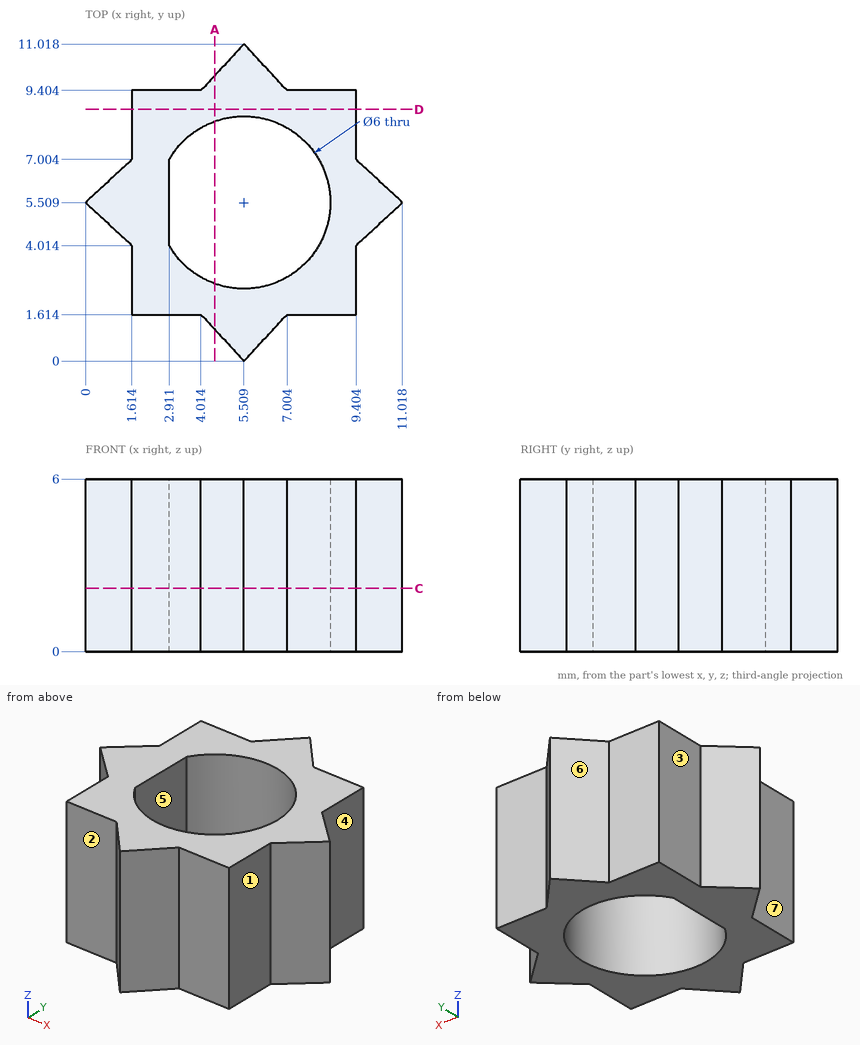
Drawing for the job (mm, zero at the part's lowest x, y, z). A direction names the side the tool comes from. Give positions to 0.01 mm unless a question says otherwise; leave off trailing zeros. Order: outer loops, then holes, each group sorted by start corner. A loop starts at its lowest first (then second) coordinate and runs counter-clockwise, first axis right, second up. Notation, with made-up numbers: (-12, 28.5) - (17, 28.5) arc R7 cw to (17, 34.5) - close; hole circle Ø1 at (56, 73.5). An arc over 180 degrees is marked (long way). Write item = value, one per line. Start each with the question number.
1. Drop flat-ended pins along their axis: P1, Ø2, axis at y = 6, z = 4, coming from the -X side; P2, Ø0.7, axis at y = 3.5, z = 2.5, coming from the -X side; P3, Ø1.9, axis at x = 2.5, z = 1.5, coming from the +Y side (1 decimal); P4, Ø1.9, axis at y = 8.5, z = 4.5, coming from the +X side (1 decimal). Give the stop position or say it passes through.
2. Probe line 1 along Y through (x, z) = (9, 4.6) (1 decimal); line 2 along X through (y, z) = (3.5, 2.75) (1 decimal); line 3 along X through (y, z) = (7.5, 4.55) (1 decimal). List the from-to ranges inside material, lowest first.
3. Cut at D-D, the plane y = 8.75. List the corners of the cut face in (x, z) (1 decimal).
4. Which spindle directions (+Z, -Z, +X, -X, +Y, -Y) get a long thin tool onto all of the face, cutting with end or side? Do the marked faces 1, 2, 3 and 4. Say none if no direction does.
5. Cut at A-A, the plane x = 4.5. List the corners of the cut face in (y, z) (1 decimal).
6. Two-plate mould, pull along Y, no slides. Class the marked faces 5, 6 and 7: pulls with the +Y half, pulls with the -Y half, needs draft (parallel to the pull), parting line crosses it, or undercut.
7. Cut at C-C, the plane z = 2.2. List the corners of the cut face in (x, y) (1 decimal).
Taken from the geometry:
q1.P1 = 0
q1.P2 = 1.61
q1.P3 = 9.4
q1.P4 = 9.4
q2.line_1 = 1.6 to 9.4
q2.line_2 = 1.6 to 3.3, 7.7 to 9.4
q2.line_3 = 1.6 to 3.3, 7.8 to 9.4
q3.outline = (1.6, 0) - (9.4, 0) - (9.4, 6) - (1.6, 6) - close
q4.face_1 = +Z, -Z, +X, -Y
q4.face_2 = +Z, -Z, -X, -Y
q4.face_3 = +Z, -Z, -X, +Y
q4.face_4 = +Z, -Z, +X, +Y
q5.outline = (1.1, 0) - (2.7, 0) - (2.7, 6) - (1.1, 6) - close; (8.3, 0) - (9.9, 0) - (9.9, 6) - (8.3, 6) - close
q6.face_5 = undercut
q6.face_6 = pulls with the +Y half
q6.face_7 = needs draft
q7.outline = (0, 5.5) - (1.6, 4) - (1.6, 1.6) - (4, 1.6) - (5.5, 0) - (7, 1.6) - (9.4, 1.6) - (9.4, 4) - (11, 5.5) - (9.4, 7) - (9.4, 9.4) - (7, 9.4) - (5.5, 11) - (4, 9.4) - (1.6, 9.4) - (1.6, 7) - close; hole (2.9, 4) arc R3 ccw (long way) to (2.9, 7) - close
